Design review of the part shown in the three views and the two pictorial views. Dimensions are in mm from the part's minimum x, y and z. Coordinates: 2 decimals unless noted, no trailing zeros. Loops run counter-clockwise (first coordinate to the right, second up) from the corner with the lowest first, then second, coordinate; pieces in that order, holes last. Notation, with made-up numbers: (-13.5, 37) -> (7.5, 37) arc R21 ccw to (7.5, 60) -> close; hole circle Ø3 at (0, 69.5). An arc over 180 degrees is marked (long way). One line per item, written item: value.
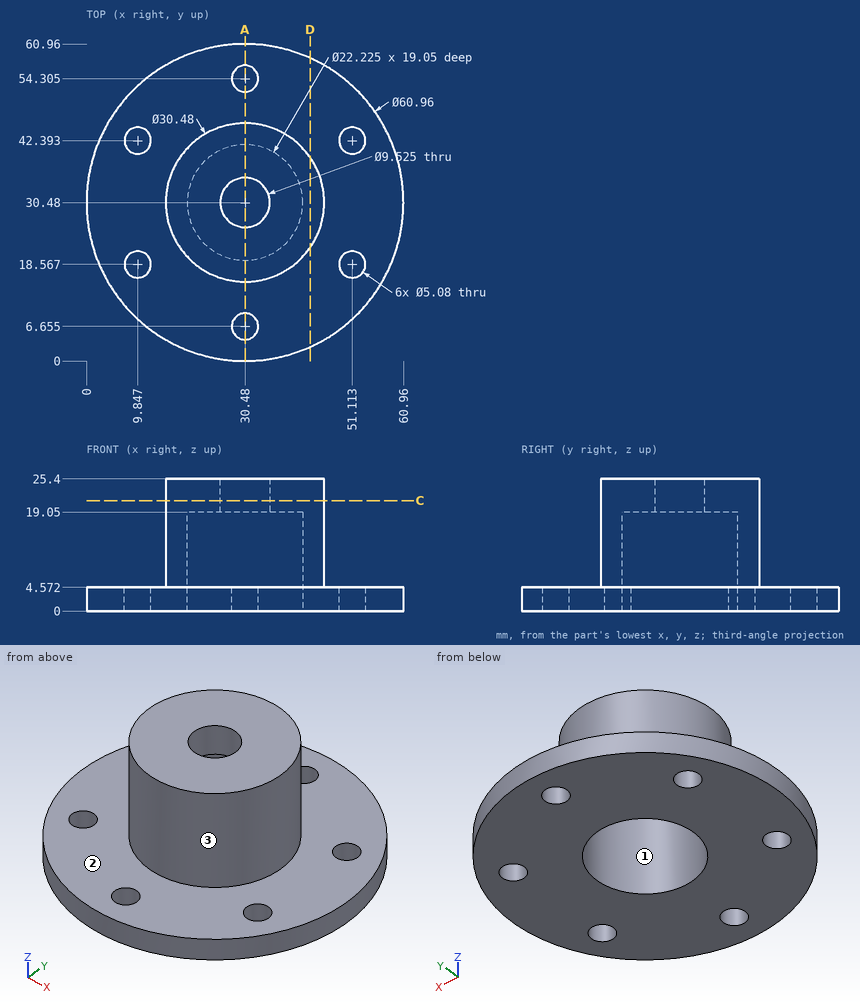
1. The part is to be moulded in two halves that separate along X. For the marked faces 1, 2 and 3, say which applies: pulls with the +X half, pulls with the -X half, needs draft (parallel to the pull), parting line crosses it, or undercut.
Return value:
face 1: undercut
face 2: needs draft
face 3: parting line crosses it
2. Take a section at D-D, the plane x = 43. Give the boundary of the cut face in (y, z).
Return value:
outline: (2.69, 0) -> (58.27, 0) -> (58.27, 4.57) -> (39.17, 4.57) -> (39.17, 25.4) -> (21.79, 25.4) -> (21.79, 4.57) -> (2.69, 4.57) -> close
3. Take a section at C-C, the plane z = 21.25. Give the boundary of the cut face in (x, y) (1 decimal).
Return value:
outline: circle Ø30.5 at (30.5, 30.5); hole circle Ø9.5 at (30.5, 30.5)
4. Insertion check: pin 1 Ø18 at (x, y) = (25, 30) entering from -Z; pin 2 Ø8 at (x, y) = (51.11, 18.57) entering from +Z; pin 3 Ø10 at (y, z) = (48.5, 13.5) entering from -X; pin 4 Ø3 at (x, z) = (28.5, 8) entering from +Y. Each pin has a flat end and moves straight along its axis. Give the tip position at first contact, or say it passes through.
Return value:
pin 1: stops at z = 0
pin 2: stops at z = 4.57
pin 3: stops at x = 22.56
pin 4: stops at y = 45.71
5. Take a section at A-A, the plane x = 30.48. Give the number of separate pieces and of enclosed holes in the cut face, and give its area (3 significant figures).
Return value:
separate pieces: 4
enclosed holes: 0
area: 383 mm2
6. To check wall thickness, follow probe 1 along Y at (x, z) = (31, 6.25); probe 2 along Y at (x, z) = (30.48, 5.5); probe 3 along Y at (x, z) = (30.48, 3.3) (1 decimal). State the ranges of each line that lie inside material, in increasing order. Write a range as from..to.
Return value:
probe 1: y = 15.25..19.38, 41.58..45.71
probe 2: y = 15.24..19.37, 41.59..45.72
probe 3: y = 0..4.1, 9.2..19.4, 41.6..51.8, 56.8..61
